from build123d import *

# Parameters (mm, degrees)
SKETCH1_W          = 19.05
SKETCH1_H          = 3.175
CHAMFER1_SIZE      = 0.9525
CUT_EXTRUDE2_DEPTH = 2.86258


with BuildPart() as part:
    # Sketch1 → Revolve1 (revolve)
    with BuildSketch(Plane(origin=(0, 0, 0), x_dir=(0, 0, -1), z_dir=(1, 0, 0))):
        with Locations((9.525, 1.5875)):
            Rectangle(SKETCH1_W, SKETCH1_H)
    revolve(axis=Axis((0, 0, -19.05), (0, 0, 1)))

    # Chamfer1
    chamfer1_edges = [part.edges().sort_by_distance(p)[0] for p in [
        (0, -3.175, -19.05),
    ]]
    chamfer(chamfer1_edges, length=CHAMFER1_SIZE)

    # Sketch7 → Revolve2 (revolve)
    with BuildSketch(Plane(origin=(0, 0, 0), x_dir=(0, 0, -1), z_dir=(1, 0, 0)), mode=Mode.PRIVATE) as revolve2_sk:
        with BuildLine():
            Line((0, 6.7437), (0.20447, 6.7437))
            Line((0.20447, 6.7437), (4.0894, 3.366581874))
            ThreePointArc((4.0894, 3.366581874), (4.328282675, 3.224461616), (4.601808997, 3.175))
            Line((4.601808997, 3.175), (4.601808997, 0))
            Line((4.601808997, 0), (0, 0))
            Line((0, 0), (0, 6.7437))
        make_face()
    revolve(revolve2_sk.sketch.rotate(Axis((0, 0, 0), (0, 0, -1)), 180), axis=Axis((0, 0, 0), (0, 0, -1)))

    # Boss-Extrude1 cone 1 section (through the dimple's axis) → Boss-Extrude1 (revolve)
    with BuildSketch(Plane(origin=(0, 0, -4.601808997), x_dir=(0, -1, 0), z_dir=(1, 0, 0))):
        Polygon((0, 0), (3.175, 0), (0, 3.06606186), align=None)
    revolve(axis=Axis((0, 0, -4.601808997), (0, 0, -1)))

    # Sketch5 → Cut-Extrude2 (cut)
    with BuildSketch(Plane.XY):
        Polygon((0, 2.291358881), (-1.984375, 1.14567944), (-1.984375, -1.14567944), (0, -2.291358881), (1.984375, -1.14567944), (1.984375, 1.14567944), align=None)
    extrude(amount=-CUT_EXTRUDE2_DEPTH, mode=Mode.SUBTRACT)

    # Cut-Extrude3 cone 1 section (through the dimple's axis) → Cut-Extrude3 (revolve, cut)
    with BuildSketch(Plane(origin=(0, 0, 0), x_dir=(0, -1, 0), z_dir=(1, 0, 0))):
        Polygon((0, 0), (2.291358881, 0), (0, 1.322916667), align=None)
    revolve(axis=Axis((0, 0, 0), (0, 0, -1)), mode=Mode.SUBTRACT)


solid = part.part
The listing builds one solid part. Answer for the finished solid, in the listing's coordinates (mm). A direction names the side the tool comes from. Round coordinates to 2 decimals unless told otherwise and drop trailing zeros. Loops run counter-clockwise (first coordinate to the right, second up) from the corner with the lowest first, then second, coordinate; pieces in that order, holes last. Notation, with made-up numbers: M 6,-18.5 L 61,-18.5 A14 ccw 61,8.5 Z; hole C 59.25,64 d6. An arc over 180 degrees is marked long. Return JSON: item names as keys, results as strings.
Q1. Find section B-B, the plane z = -13. Determine the outline of the cut face in (x, y) (3 decimals), plus the area to 3 significant figures.
Results list:
{"outline": "C 0,0 d6.35", "area": "31.7 mm2"}
Q2. Each of these flat-tipped pins is pushed along its axis until it touches: pin 1 Ø1.8 at (y, z) = (-0.5, -1.5) entering from +X; pin 2 Ø2 at (x, z) = (-1, -9.5) entering from +Y (3 decimals); pin 3 Ø2.5 at (y, z) = (0, -1.5) entering from -X. Where does it stop, or does it pass through?
Results list:
{"pin 1": "stops at x = 6.38", "pin 2": "stops at y = 3.175", "pin 3": "stops at x = -6.7"}
Q3. Which of the six approach directions +Z, -Z, +X, -X, +Y, -Y give full straight-line access (tool end or side, diameter ignored) to faces 1 (the face through (3.1, -0.69, -11.44)), 2 (the face through (-0.978, 1.727, -1.411)), 3 (the face through (0, 3, 0))?
Results list:
{"face 1": "-Z", "face 2": "+Z", "face 3": "+Z, +X, -X, +Y, -Y"}
Q4. The mould has two halves that part along Y. Classify faces 4 (the face through (1.01, 1.71, -1.41)), 5 (the face through (0, 0, -19.05)), 6 (the face through (3.13, -1.63, -3.9)): released by +Y, released by -Y, zero draft, split by the parting line, or undercut.
Results list:
{"face 4": "undercut", "face 5": "zero draft", "face 6": "split by the parting line"}
Q5. Find the intervals of material crossed by line 1 along X through (y, z) = (0, -9.5) (3 decimals); line 2 along X through (y, z) = (-1.25, -2.5); line 3 along Z through (x, y) = (-1, -0.25), in increasing order. Write a range as from..to.
Results list:
{"line 1": "x = -3.175..3.175", "line 2": "x = -4.58..-1.8, 1.8..4.58", "line 3": "z = -19.05..-2.86"}
